Read the model definition and answer for the solid it produces. Units are mm, in the model's axes. A direction names the side the tool comes from. Coordinates: 2 decimals unless noted, no trailing zeros. Order: outer loops, then holes, each group sorted by start corner. A loop starts at its lowest first (then second) coordinate and runs counter-clockwise, first axis right, second up. Notation, with made-up numbers: (40.25, -22) -> (59.25, -22) arc R22 ccw to (59.25, -3) -> close; hole circle Ø3 at (-19, 77.25). An arc over 180 degrees is marked (long way). Return JSON: item names as keys, results as strings. Group by question number.
```python
from build123d import *

# Parameters (mm, degrees)
BOSS_EXTRUDE1_DEPTH = 31.2
BOSS_EXTRUDE2_DEPTH = 10
CUT_EXTRUDE1_START  = -31.2
SKETCH6_R           = 1.6999999999999995
CUT_EXTRUDE1_DEPTH  = 31.2
CUT_EXTRUDE2_DEPTH  = 3.25
CHAMFER1_SIZE       = 1.75
FILLET2_R           = 4
CUT_EXTRUDE3_DEPTH  = 7.5


with BuildPart() as part:
    # Sketch4 → Boss-Extrude1 (new body)
    with BuildSketch(Plane(origin=(15.600000000000225, 5.91e-15, 1.0893e-13), x_dir=(3.8e-16, -1, 0), z_dir=(-1, -3.8e-16, -6.98e-15))):
        Polygon((12.836171405416206, 32.32337770791894), (-3.4906338806220005, 51.78090656314089), (-5.485895724995086, 32.32337770791894), align=None)
    extrude(amount=BOSS_EXTRUDE1_DEPTH)

    # Sketch5 → Boss-Extrude2 (add)
    with BuildSketch(Plane(origin=(-2.2571e-13, 0, 32.323377707918944), x_dir=(-1, 0, -6.98e-15), z_dir=(6.98e-15, 0, -1))):
        Polygon((-15.600000000000223, 5.485895724995093), (-15.60000000000023, -12.8361714054162), (15.599999999999769, -12.836171405416213), (15.599999999999776, 5.485895724995081), align=None)
        Polygon((-12.725000000000225, -11.125000000000004), (-9.475000000000225, -11.125000000000004), (-9.475000000000227, 3.1250000000000013), (-12.725000000000227, 3.125000000000001), align=None, mode=Mode.SUBTRACT)
        Polygon((12.724999999999774, -11.125000000000002), (9.474999999999774, -11.125), (9.474999999999772, 3.1250000000000018), (12.724999999999772, 3.1250000000000027), align=None, mode=Mode.SUBTRACT)
    extrude(amount=BOSS_EXTRUDE2_DEPTH)

    # Sketch6 → Cut-Extrude1 (cut)
    with BuildSketch(Plane(origin=(15.600000000000225, 5.91e-15, 1.0909e-13), x_dir=(6.99e-15, 0, -1), z_dir=(1, 3.8e-16, 6.99e-15)).offset(CUT_EXTRUDE1_START)):
        with Locations((-27.32337770791874, -4.000000000000007)):
            Circle(SKETCH6_R)
    extrude(amount=CUT_EXTRUDE1_DEPTH, mode=Mode.SUBTRACT)

    # Sketch8 → Cut-Extrude2 (cut)
    with BuildSketch(Plane(origin=(9.475000000000227, -1.15e-15, 6.616e-14), x_dir=(6.98e-15, 0, -1), z_dir=(1, 0, 6.98e-15))):
        Polygon((-32.323377707918944, -11.125000000000002), (-32.323377707918944, 3.1250000000000027), (-39.44837770791897, -3.999999999999999), align=None)
    cut_extrude2 = extrude(amount=CUT_EXTRUDE2_DEPTH, mode=Mode.SUBTRACT)

    # Chamfer1
    chamfer1_edges = [part.edges().sort_by_distance(p)[0] for p in [
        (-15.599999999999975, -4.000000000000013, 29.02337770791863),
        (15.600000000000025, -4.000000000000001, 29.02337770791885),
    ]]
    chamfer(chamfer1_edges, length=CHAMFER1_SIZE)

    # Mirror1: Cut-Extrude2 across plane
    add(cut_extrude2.mirror(Plane(origin=(0, 0, 0), x_dir=(0, 0, 1), z_dir=(1, 0, 0))), mode=Mode.SUBTRACT)

    # Fillet2
    # the kernel refuses this fillet: 4 mm, written as the material it takes off along each edge
    with BuildSketch(Plane(origin=(-15.600000000000204, 2.4705385648813603, 61.72874077701889), x_dir=(1, 3.9e-16, 6.98e-15), z_dir=(6.907902673272719e-15, 0.10200953157406341, -0.9947834213878116))) as fillet2_piece_1:
        with BuildLine():
            CenterArc((FILLET2_R, FILLET2_R), FILLET2_R, 180, 90)
            Line((2.72e-15, FILLET2_R), (0, 0))
            Line((0, 0), (FILLET2_R, 0))
        make_face()
    extrude(amount=39.55956285246186, mode=Mode.SUBTRACT)
    with BuildSketch(Plane(origin=(16.11138148873873, 5.485895724995093, 32.323377707919036), x_dir=(-6.90790267327272e-15, -0.10200953157406191, 0.9947834213878117), z_dir=(-1, -3.8e-16, -6.98e-15))) as fillet2_piece_2:
        with BuildLine():
            CenterArc((FILLET2_R * 0.0511381488739, -FILLET2_R), FILLET2_R, 89.9999999999999, 5.854900023063593)
            Line((-FILLET2_R * 0.0508713827002, -FILLET2_R * 0.00521657861219), (0, 0))
            Line((0, 0), (FILLET2_R * 0.0511381488739, 0))
        make_face()
    extrude(amount=32.22276297747746, mode=Mode.SUBTRACT)
    with BuildSketch(Plane(origin=(15.599999999999794, 2.470538564881372, 61.72874077701911), x_dir=(0, -0.9947834213878115, -0.1020095315740634), z_dir=(6.907902673272719e-15, 0.10200953157406341, -0.9947834213878116))) as fillet2_piece_3:
        with BuildLine():
            CenterArc((FILLET2_R, FILLET2_R), FILLET2_R, 180, 90)
            Line((6.7e-16, FILLET2_R), (0, 0))
            Line((0, 0), (FILLET2_R, 0))
        make_face()
    extrude(amount=39.559562852461866, mode=Mode.SUBTRACT)

    # Sketch9 → Cut-Extrude3 (cut)
    with BuildSketch(Plane.XY.offset(32.32337770791894)):
        with BuildLine():
            Line((3, 5.485895724995084), (5.5, 5.485895724995082))
            ThreePointArc((5.5, 5.485895724995082), (-1.4e-15, -0.01410427500491185), (-5.5, 5.485895724995082))
            Line((-5.5, 5.485895724995082), (-3, 5.485895724995084))
            ThreePointArc((-3, 5.485895724995084), (-1.55e-15, 2.485895724995088), (3, 5.485895724995084))
        make_face()
    extrude(amount=CUT_EXTRUDE3_DEPTH, mode=Mode.SUBTRACT)


solid = part.part
```
1. Find section A-A on x = 9. Determine the outline of the cut face in (y, z), and give its area (3 significant figures).
2. Find section D-D on z = 36. Give the number of separate pieces and of enclosed holes in the cut face, and give its area (3 significant figures).
3. For a pull along Z with two mould halves and no side action, classify faces 4 (the face through (14.4, 3.84, 37.19)), 5 (the face through (-9.475, -3, 29)), 6 (the face through (-13.295, -4.651, 25.753)) as released by +Z, released by -Z, zero draft, split by the parting line, or undercut.
4. Find section C-C on y = -8. Determine the outline of the cut face in (x, z) (3 decimals).
5. Find section B-B on x = 0. Determine the outline of the cut face in (y, z), and give its area (3 significant figures).
6. Given pin 1 (3 mm diameter, centred on y = -4, z = 27.32, fed in from -X); pin 2 (10 mm diameter, centred on x = 5.5, y = 3.5, fed in from +Z); pin 3 (1.5 mm diameter, centred on x = 11.5, y = -9.5, fed in from -Z); pin 4 (2 mm diameter, centred on x = -9.5, y = -8.5, fed in from +Z), each flat-ended and moving along its own axis, determine where each tip first touches the part or whether it passes through.
7. Straight lines are drawn through the part: L1, parallel to X at y = -5, z = 31.5 (3 decimals); L2, parallel to X at y = -6.75, z = 26.75 (3 decimals); L3, parallel to Z at x = 1.5, y = -4. For each, find the intervals that lie inside material, in ascending order.
8. Which of the six approach directions +Z, -Z, +X, -X, +Y, -Y give full straight-line access (tool end or side, diameter ignored) to faces 1 (the face through (-11.08, -7.51, 35.94)), 2 (the face through (0, 2, 39.823)), 3 (the face through (13.3, -3.5, 25.7))?
Result:
{
 "1": {"outline": "(-12.84, 22.32) -> (5.49, 22.32) -> (5.49, 32.12) arc R4 ccw to (5.47, 32.53) -> (3.49, 51.78) -> (-12.84, 32.32) -> close; hole circle Ø3.4 at (-4, 27.32)", "area": "352 mm^2"},
 "2": {"separate pieces": "2", "enclosed holes": "2", "area": "380 mm^2"},
 "3": {"face 4": "released by +Z", "face 5": "zero draft", "face 6": "undercut"},
 "4": {"outline": "(-15.6, 22.323) -> (-12.725, 22.323) -> (-12.725, 35.448) -> (-9.475, 35.448) -> (-9.475, 22.323) -> (9.475, 22.323) -> (9.475, 35.448) -> (12.725, 35.448) -> (12.725, 22.323) -> (15.6, 22.323) -> (15.6, 38.087) -> (-15.6, 38.087) -> close"},
 "5": {"outline": "(-12.84, 22.32) -> (5.49, 22.32) -> (5.49, 32.12) arc R4 ccw to (5.47, 32.53) -> (3.49, 51.78) -> (-12.84, 32.32) -> close; hole circle Ø3.4 at (-4, 27.32); hole (-0.01, 32.32) -> (2.49, 32.32) -> (2.49, 39.82) -> (-0.01, 39.82) -> close", "area": "334 mm^2"},
 "6": {"pin 1": "through", "pin 2": "z = 51.78", "pin 3": "z = 33.2", "pin 4": "z = 38.68"},
 "7": {"L1": "-15.6 to -12.725, -9.475 to 9.475, 12.725 to 15.6", "L2": "-14.959 to -12.725, -9.475 to 9.475, 12.725 to 14.959", "L3": "22.32 to 25.62, 29.02 to 42.85"},
 "8": {"face 1": "-Z", "face 2": "none", "face 3": "+X, -X"}
}
